Autodesk Inventor part; units mm, degrees
ref_plane "YZ Plane" through (0, 0, 0) normal (1, 0, 0) x (0, 1, 0)
ref_plane "XZ Plane" through (0, 0, 0) normal (0, 1, 0) x (-1, 0, 0)
ref_plane "XY Plane" through (0, 0, 0) normal (0, 0, 1) x (1, 0, 0)
sketch "Sketch1" plane through (0, 0, 0) normal (1, 0, 0) x (0, 1, 0)
  circle A0 centre (0, 0) radius 8.509
  dimension "d1" = 17.018
extrude "Extrusion1" add sketch "Sketch1" along normal blind 2.54
sketch "Sketch2" plane through (2.54, 0, 0) normal (1, 0, 0) x (0, 0, -1)
  circle A0 centre (0, 0) radius 8.509
  circle A1 centre (0, 0) radius 4.0005
  dimension "d5" = 8.001
extrude "Extrusion2" add sketch "Sketch2" along normal blind 6.096 contours A1
sketch "Sketch3" plane through (0, 0, 0) normal (-1, 0, 0) x (0, 0, 1)
  circle A0 centre (0, 0) radius 8.509
  circle A1 centre (6.9342, 0) radius 1.5875
  line L0 (6.9342, -1.5875) -> (8.3596, -1.5875)
  line L1 (6.9342, 1.5875) -> (8.3596, 1.5875)
  line L2 (6.9342, 0) -> (0, 0)
  dimension "d8" = 6.9342
  dimension "d9" = 3.175
extrude "Extrusion3" cut sketch "Sketch3" against normal through all contours A0 A1 L1 | L0 A1 A0 | A1 A0 | A0 A1
properties part number "Pulley Shaft" material "Steel"
Build history of the part. All positions in model axes, mm. A direction names the side the tool comes from. Coordinates: 2 decimals unless noted, no trailing zeros. Write each loop counter-clockwise with the first axis right and the second up, starting at its lowest first coordinate (ties: lowest second). Pieces come first, ordered by that corner, then holes.
(1) Cut at D-D on z = -5.75. List the corners of the cut face in (x, y), and give its area (3 significant figures).
(2) Drill centre lines: line 1 (X direction, y = 4, z = 0.75); line 2 (Y direction, x = 6.5, z = -2.25); line 3 (Y direction, x = 1, z = -2.75). Where is each one in solid material? Low to high.
(3) Cut at B-B on y = 0. List the corners of the cut face in (x, z), and give its area (3 significant figures).
(4) Mould opens along Y. For faces 4 (the cylindrical face through (5.5, 3.9, 0.9)), 5 (the flat face through (0, 0, 0)), 6 (the flat face through (1, -1.588, 8)) say: pulls with the +Y half, pulls with the -Y half, needs draft (parallel to the pull), parting line crosses it, or undercut.
(5) Pin check, flat tips, straight feed: pin 1 Ø4 at (x, y) = (2, -1.5) entering from +Z; pin 2 Ø0.7 at (x, z) = (2, 7.5) entering from +Y; pin 3 Ø3 at (x, z) = (1.5, 5) entering from +Y; pin 4 Ø1.5 at (x, y) = (8, 0) entering from +Z. Stop position of each tip, or through.
(6) 3-axis set-ups, long thin cutter, end or side, ignore diameter. For faces 1 (the flat face through (1, 1.588, 8)), 2 (the flat face through (2.54, 2, -4)), 3 (the flat face through (8.636, 0, 0)): which of +Z, -Z, +X, -X, +Y, -Y reach the whole face in a straight line?
(7) Cut at A-A on z = 0. List the corners of the cut face in (x, y), and give its area (3 significant figures).
(8) Cut at C-C on x = 2.25. List the corners of the cut face in (y, z) (1 decimal), and give its area (3 significant figures).
Working result:
1. outline: (0, -6.27) - (2.54, -6.27) - (2.54, 6.27) - (0, 6.27) - close
1. area: 31.9 mm2
2. line 1: x = 0 to 2.54
2. line 2: y = -3.31 to 3.31
2. line 3: y = -8.05 to 8.05
3. outline: (0, -8.51) - (2.54, -8.51) - (2.54, -4) - (8.64, -4) - (8.64, 4) - (2.54, 4) - (2.54, 5.35) - (0, 5.35) - close
3. area: 84.0 mm2
4. face 4: parting line crosses it
4. face 5: needs draft
4. face 6: undercut
5. pin 1: stops at z = 8.36
5. pin 2: stops at y = 4.61
5. pin 3: stops at y = 7.76
5. pin 4: stops at z = 4
6. face 1: +Z, +X, -X
6. face 2: +X
6. face 3: +Z, -Z, +X, +Y, -Y
7. outline: (0, -8.51) - (2.54, -8.51) - (2.54, -4) - (8.64, -4) - (8.64, 4) - (2.54, 4) - (2.54, 8.51) - (0, 8.51) - close
7. area: 92.0 mm2
8. outline: (-1.6, 6.9) - (-1.6, 8.4) arc R8.5 ccw (long way) to (1.6, 8.4) - (1.6, 6.9) arc R1.6 cw to start
8. area: 219 mm2
